Read the model definition and answer for the solid it produces. Units are mm, in the model's axes. A direction names the side the tool comes from. Coordinates: 2 decimals unless noted, no trailing zeros. Order: outer loops, then holes, each group sorted by start corner. A loop starts at its lowest first (then second) coordinate and runs counter-clockwise, first axis right, second up. Notation, with made-up numbers: (7, 19) -> (24, 19) arc R10 cw to (24, 33) -> close; hole circle Ø2 at (31.25, 37). An arc over 180 degrees is marked (long way). Answer as a JSON object with one key per item and string values. Group by question number.
1) Section B-B on x = -37.5 is taken. Determine the outline of the cut face in (y, z).
2) Determine the mould class of faces 5 (the flat face through (34, -21, 16)), 6 (the cylindrical face through (21.634, 36.426, 2.986)), 7 (the cylindrical face through (-57.524, -32.602, 0.986)) for opening direction Y: released by +Y, released by -Y, zero draft, split by the parting line, or undercut.
3) Given pin 1 (6 mm diameter, centred on y = 7, z = 3.5, fed in from -X); pin 2 (9 mm diameter, centred on x = 40, y = -21, fed in from -Z); pin 3 (5 mm diameter, centred on x = -19.5, y = 54, fed in from +Z); pin 4 (6 mm diameter, centred on y = 55, z = 6.5, fed in from -X), each flat-ended and moving along its own axis, determine where each tip first touches the part or whether it passes through.
4) A tool of negligible diameter and unlimited length cuts with its end or side. For faces 1 (the cylindrical face through (-41.035, -28.666, 9.916)), 2 (the cylindrical face through (-35.39, 20.7, 2.99)), 3 (the cylindrical face through (35.62, 20.3, 2.99)), 4 (the cylindrical face through (-21.593, 36.538, 2.986)), from which of +Z, -Z, +X, -X, +Y, -Y can it reach the whole face along a straight path? Write none if from no direction.
5) Section C-C on x = 50.5 is taken. Determine the outline of the cut face in (y, z).
6) Section A-A on z = 10.5 is taken. Determine the outline of the cut face in (x, y), and give its area (3 significant figures).
7) Section D-D on y = 12.5 is taken. Determine the outline of the cut face in (x, z).
8) Consider L1, parallel to X at y = -23.5, z = 8.25; L2, parallel to X at y = -24, z = 0.75; L3, parallel to Z at x = 17, y = -34.5. Determine where each line is inside the solid, lowest interval first.
from build123d import *

# Parameters (mm, degrees)
SKETCH1_R           = 5.5
BOSS_EXTRUDE1_DEPTH = 4
CUT_EXTRUDE1_START  = -2
CUT_EXTRUDE1_DEPTH  = 2
SKETCH4_R           = 8
BOSS_EXTRUDE2_DEPTH = 16
SKETCH6_R           = 3
CUT_EXTRUDE2_DEPTH  = 4
SKETCH7_R           = 5.5
CUT_EXTRUDE3_DEPTH  = 91.325305156


with BuildPart() as part:
    # Sketch1 → Boss-Extrude1 (new body)
    with BuildSketch(Plane.XY):
        with BuildLine():
            ThreePointArc((22.877204778, 40.819588003), (-0.010726273, 66.124665414), (-22.890446501, 40.812163899))
            ThreePointArc((-22.890446501, 40.812163899), (-23.449446231, 37.285381871), (-25.675278589, 34.493188739))
            ThreePointArc((-25.675278589, 34.493188739), (-37.24257945, 21.493959056), (-42.711233264, 4.974992775))
            ThreePointArc((-42.711233264, 4.974992775), (-44.015348899, 1.650845578), (-46.789402571, -0.597553496))
            ThreePointArc((-46.789402571, -0.597553496), (-57.260276929, -33.071621932), (-23.89914747, -40.229790123))
            ThreePointArc((-23.89914747, -40.229790123), (-20.565364774, -38.950507076), (-17.034338411, -39.482037877))
            ThreePointArc((-17.034338411, -39.482037877), (0.006975154, -42.999999434), (17.047146505, -39.476509421))
            ThreePointArc((17.047146505, -39.476509421), (20.578000241, -38.943833092), (23.912197793, -40.222034507))
            ThreePointArc((23.912197793, -40.222034507), (57.271003202, -33.053043482), (46.789593971, -0.582373776))
            ThreePointArc((46.789593971, -0.582373776), (44.014811006, 1.665125206), (42.709617, 4.988849138))
            ThreePointArc((42.709617, 4.988849138), (37.235604296, 21.506040378), (25.664086758, 34.501516646))
            ThreePointArc((25.664086758, 34.501516646), (23.437348658, 37.292987514), (22.877204778, 40.819588003))
        make_face()
        with Locations((-0.006995377, 43.124665717)):
            Circle(SKETCH1_R, mode=Mode.SUBTRACT)
        with Locations((37.350553729, -21.556274684)):
            Circle(SKETCH1_R, mode=Mode.SUBTRACT)
        with Locations((-37.343558352, -21.568391032)):
            Circle(SKETCH1_R, mode=Mode.SUBTRACT)
    extrude(amount=BOSS_EXTRUDE1_DEPTH)

    # Sketch2 → Cut-Extrude1 (cut)
    with BuildSketch(Plane.XY.offset(4).offset(CUT_EXTRUDE1_START)):
        with BuildLine():
            ThreePointArc((22.877204778, 40.819588003), (23.437348658, 37.292987514), (25.664086758, 34.501516646))
            ThreePointArc((25.664086758, 34.501516646), (37.235604296, 21.506040378), (42.709617, 4.988849138))
            ThreePointArc((42.709617, 4.988849138), (44.014811006, 1.665125206), (46.789593971, -0.582373776))
            ThreePointArc((46.789593971, -0.582373776), (57.271003202, -33.053043482), (23.912197793, -40.222034507))
            ThreePointArc((23.912197793, -40.222034507), (20.578000241, -38.943833092), (17.047146505, -39.476509421))
            ThreePointArc((17.047146505, -39.476509421), (0.006975154, -42.999999434), (-17.034338411, -39.482037877))
            ThreePointArc((-17.034338411, -39.482037877), (-20.565364774, -38.950507076), (-23.89914747, -40.229790123))
            ThreePointArc((-23.89914747, -40.229790123), (-57.260276929, -33.071621932), (-46.789402571, -0.597553496))
            ThreePointArc((-46.789402571, -0.597553496), (-44.015348899, 1.650845578), (-42.711233264, 4.974992775))
            ThreePointArc((-42.711233264, 4.974992775), (-37.24257945, 21.493959056), (-25.675278589, 34.493188739))
            ThreePointArc((-25.675278589, 34.493188739), (-23.449446231, 37.285381871), (-22.890446501, 40.812163899))
            ThreePointArc((-22.890446501, 40.812163899), (-0.010726273, 66.124665414), (22.877204778, 40.819588003))
        make_face()
        with BuildLine():
            ThreePointArc((-24.481079585, 32.888854379), (-35.510366452, 20.49424003), (-40.724664275, 4.743597762))
            ThreePointArc((-40.724664275, 4.743597762), (-42.401384377, 0.469694224), (-45.968024813, -2.421104586))
            ThreePointArc((-45.968024813, -2.421104586), (-55.528388357, -32.071340985), (-25.068226677, -38.607059768))
            ThreePointArc((-25.068226677, -38.607059768), (-20.78193464, -36.962267279), (-16.242043601, -37.645664022))
            ThreePointArc((-16.242043601, -37.645664022), (0.006650729, -40.999999461), (16.25425597, -37.640392703))
            ThreePointArc((16.25425597, -37.640392703), (20.793925059, -36.955523138), (25.080750483, -38.598924957))
            ThreePointArc((25.080750483, -38.598924957), (55.538790204, -32.053324456), (45.968807863, -2.406191246))
            ThreePointArc((45.968807863, -2.406191246), (42.401229765, 0.483450301), (40.723123186, 4.756809644))
            ThreePointArc((40.723123186, 4.756809644), (35.503715724, 20.50575943), (24.470408304, 32.896794941))
            ThreePointArc((24.470408304, 32.896794941), (21.607459318, 36.485828914), (20.88727433, 41.020029543))
            ThreePointArc((20.88727433, 41.020029543), (-0.010401848, 64.12466544), (-20.900581186, 41.013251014))
            ThreePointArc((-20.900581186, 41.013251014), (-21.619295125, 36.478816977), (-24.481079585, 32.888854379))
        make_face(mode=Mode.SUBTRACT)
    extrude(amount=CUT_EXTRUDE1_DEPTH, mode=Mode.SUBTRACT)

    # Sketch4 → Boss-Extrude2 (add)
    with BuildSketch(Plane(origin=(0, 0, 0), x_dir=(-1, 0, 0), z_dir=(0, 0, -1))):
        with Locations((0.006995377, 43.124665717)):
            Circle(SKETCH4_R)
        with Locations((-37.350553729, -21.556274684)):
            Circle(SKETCH4_R)
        with Locations((37.343558352, -21.568391032)):
            Circle(SKETCH4_R)
    extrude(amount=-BOSS_EXTRUDE2_DEPTH)

    # Sketch6 → Cut-Extrude2 (cut)
    with BuildSketch(Plane.XY.offset(16)):
        with Locations((-0.006995377, 43.124665717)):
            Circle(SKETCH6_R)
        with Locations((-37.343558352, -21.568391032)):
            Circle(SKETCH6_R)
        with Locations((37.350553729, -21.556274684)):
            Circle(SKETCH6_R)
    extrude(amount=-CUT_EXTRUDE2_DEPTH, mode=Mode.SUBTRACT)

    # Sketch7 → Cut-Extrude3 (cut, through all)
    with BuildSketch(Plane.XY.offset(12)):
        with Locations((-0.006995377, 43.124665717)):
            Circle(SKETCH7_R)
        with Locations((-37.343558352, -21.568391032)):
            Circle(SKETCH7_R)
        with Locations((37.350553729, -21.556274684)):
            Circle(SKETCH7_R)
    extrude(amount=-CUT_EXTRUDE3_DEPTH, mode=Mode.SUBTRACT)


solid = part.part
Worked answers:
{
 "1": {"outline": "(-44.57, 0) -> (-27.07, 0) -> (-27.07, 12) -> (-24.56, 12) -> (-24.56, 16) -> (-29.57, 16) -> (-29.57, 4) -> (-42.57, 4) -> (-42.57, 2) -> (-44.57, 2) -> close; (-18.57, 12) -> (-16.07, 12) -> (-16.07, 0) -> (21.04, 0) -> (21.04, 2) -> (16.58, 2) -> (16.58, 4) -> (-13.57, 4) -> (-13.57, 16) -> (-18.57, 16) -> close"},
 "2": {"face 5": "zero draft", "face 6": "undercut", "face 7": "split by the parting line"},
 "3": {"pin 1": "stops at x = -42.8", "pin 2": "stops at z = 0", "pin 3": "stops at z = 4", "pin 4": "stops at x = -18.35"},
 "4": {"face 1": "+Z", "face 2": "+Z, -X, +Y", "face 3": "+Z, +X, +Y", "face 4": "+Z, -X"},
 "5": {"outline": "(-40.43, 0) -> (-2.69, 0) -> (-2.69, 2) -> (-5.18, 2) -> (-5.18, 4) -> (-37.93, 4) -> (-37.93, 2) -> (-40.43, 2) -> close"},
 "6": {"outline": "circle Ø16 at (-37.34, -21.57); circle Ø16 at (-0.01, 43.12); circle Ø16 at (37.35, -21.56); hole circle Ø11 at (-37.34, -21.57); hole circle Ø11 at (-0.01, 43.12); hole circle Ø11 at (37.35, -21.56)", "area": "318 mm²"},
 "7": {"outline": "(-41.14, 0) -> (41.14, 0) -> (41.14, 2) -> (39.05, 2) -> (39.05, 4) -> (-39.05, 4) -> (-39.05, 2) -> (-41.14, 2) -> close"},
 "8": {"L1": "x = -45.11 to -42.49, -32.19 to -29.58, 29.59 to 32.21, 42.5 to 45.11", "L2": "x = -60.21 to -42.28, -32.41 to 32.42, 42.28 to 60.22", "L3": "z = 0 to 4"}
}
